Could you check a few things on this model? Use its own coordinates, in mm. Coordinates: 2 decimals unless noted, no trailing zeros. Loops run counter-clockwise (first coordinate to the right, second up) from the corner with the lowest first, then second, coordinate; pieces in that order, holes last.
from build123d import *

# Parameters (mm, degrees)
F0_R     = 13.335
F1_DEPTH = 6.35


with BuildPart() as f1:
    # F0 (on Top) → F1 (new body)
    with BuildSketch(Plane.XY):
        with BuildLine():
            Line((0, 0), (0, 15.875))
            ThreePointArc((0, 15.875), (-27.10032, 27.10032), (-15.875, 0))
            Line((-15.875, 0), (0, 0))
        make_face()
        with Locations((-15.875, 15.875)):
            Circle(F0_R, mode=Mode.SUBTRACT)
    extrude(amount=F1_DEPTH)

    # F2: F1 across plane


with BuildPart() as f1_1:
    add(f1.part)
    add(f1.part.mirror(Plane.YZ))

    # F3: F1 across plane


with BuildPart() as f1_2:
    add(f1_1.part)
    add(f1_1.part.mirror(Plane.XZ))


solid = f1_2.part
1) Imagine slicing it at B-B on y = 22.5. List the corners of the cut face in (x, z) for me, plus the area to 3 significant figures.
2) If I drill on L1, parallel to X at y = 5, z = 4.25; L2, parallel to Y at x = -28, z = 1.75; L3, parallel to Y at x = 4, z = 2.75, over which ranges is the centre line in solid material (lowest first)?
3) Imagine slicing it at C-C on x = 8.5. List the corners of the cut face in (y, z) for me, plus the area to 3 significant figures.
4) Imagine slicing it at A-A on x = -24. List the corners of the cut face in (y, z) for me, plus the area to 3 significant figures.
5) We'd pull the mould along X, two halves only. Please class faces 1 (the cylindrical face through (17.611, 29.097, 3.131)), 2 (the flat face through (3, -3, 6.35)): released by +X, released by -X, zero draft, split by the parting line, or undercut.
6) Imagine slicing it at D-D on z = 1.75. List the corners of the cut face in (x, y) for me (3 decimals), plus the area to 3 significant figures.
7) Will these pins go through, and if not, where does the flat tip stop? pin 1 (2 mm diameter, centred on y = -11, z = 2, fed in from +X); pin 2 (24 mm diameter, centred on x = -15.875, y = 15.875, fed in from -Z).
Solved:
1. outline: (-30.3, 0) - (-27.45, 0) - (-27.45, 6.35) - (-30.3, 6.35) - close; (-4.3, 0) - (-1.45, 0) - (-1.45, 6.35) - (-4.3, 6.35) - close; (1.45, 0) - (4.3, 0) - (4.3, 6.35) - (1.45, 6.35) - close; (27.45, 0) - (30.3, 0) - (30.3, 6.35) - (27.45, 6.35) - close
1. area: 72.5 mm2
2. L1: x = -27.44 to -23.59, -8.16 to 8.16, 23.59 to 27.44
2. L2: y = -26.12 to -21.43, -10.32 to -5.63, 5.63 to 10.32, 21.43 to 26.12
2. L3: y = -26.41 to -21.94, -9.81 to 9.81, 21.94 to 26.41
3. outline: (-29.93, 0) - (-26.98, 0) - (-26.98, 6.35) - (-29.93, 6.35) - close; (-4.77, 0) - (4.77, 0) - (4.77, 6.35) - (-4.77, 6.35) - close; (26.98, 0) - (29.93, 0) - (29.93, 6.35) - (26.98, 6.35) - close
3. area: 98.0 mm2
4. outline: (-29.51, 0) - (-26.45, 0) - (-26.45, 6.35) - (-29.51, 6.35) - close; (-5.3, 0) - (-2.24, 0) - (-2.24, 6.35) - (-5.3, 6.35) - close; (2.24, 0) - (5.3, 0) - (5.3, 6.35) - (2.24, 6.35) - close; (26.45, 0) - (29.51, 0) - (29.51, 6.35) - (26.45, 6.35) - close
4. area: 77.8 mm2
5. face 1: undercut
5. face 2: zero draft
6. outline: (-15.875, 0) arc R15.875 ccw (long way) to (0, -15.875) arc R15.875 ccw (long way) to (15.875, 0) arc R15.875 ccw (long way) to (0, 15.875) arc R15.875 ccw (long way) to start; hole circle Ø26.67 at (-15.875, -15.875); hole circle Ø26.67 at (-15.875, 15.875); hole circle Ø26.67 at (15.875, -15.875); hole circle Ø26.67 at (15.875, 15.875)
6. area: 1,150 mm2
7. pin 1: stops at x = 31.27
7. pin 2: passes through
